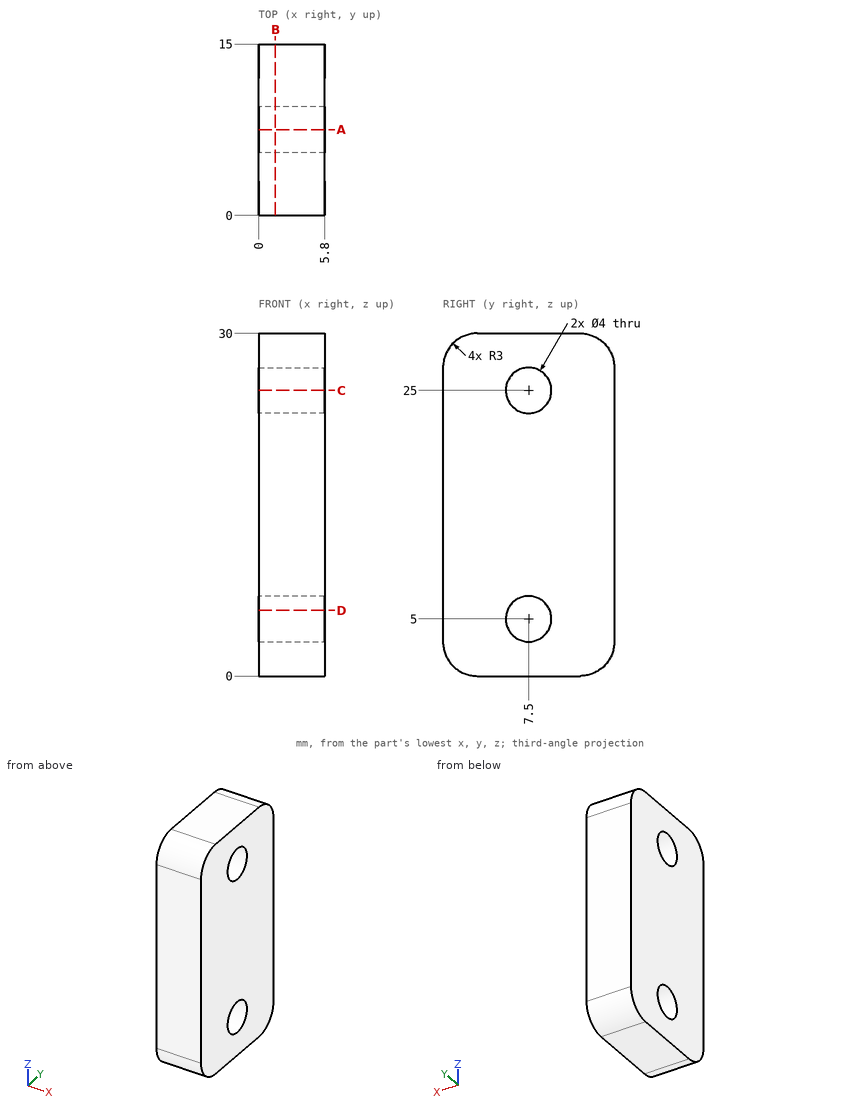
Print and shaded views of the part. All mm, measured from the part's lowest x, y and z. Round coordinates to 2 decimals unless told otherwise and drop trailing zeros. Loops run counter-clockwise (first coordinate to the right, second up) from the corner with the lowest first, then second, coordinate; pieces in that order, holes last. Notation, with made-up numbers: (7, 46) -> (65, 46) arc R20 ccw to (65, 71) -> close; hole circle Ø2 at (34, 47.5). An arc over 180 degrees is marked (long way). Use CSV: the item, a comma, the result in double quotes. Start each with the question number.
1) Wall check: L1, parallel to Y at x = 1.45, z = 5; L2, parallel to Z at x = 1.1, y = 9; L3, parallel to Z at x = 3.75, y = 6.5. Give the ranges that are in metal, low to high. Write a range as [from, to].
2) Cut at A-A, the plane y = 7.5. Write the cut outline in (x, z).
3) Cut at D-D, the plane z = 5.75. Write the cut outline in (x, y).
4) Cut at B-B, the plane x = 1.45. Write the cut outline in (y, z), plus the area to 3 significant figures.
5) Cut at C-C, the plane z = 25. Write the cut outline in (x, y), plus the area to 3 significant figures.
Determined:
1,L1,"y = [0, 5.5], [9.5, 15]"
1,L2,"z = [0, 3.68], [6.32, 23.68], [26.32, 30]"
1,L3,"z = [0, 3.27], [6.73, 23.27], [26.73, 30]"
2,outline,"(0, 0) -> (5.8, 0) -> (5.8, 3) -> (0, 3) -> close; (0, 7) -> (5.8, 7) -> (5.8, 23) -> (0, 23) -> close; (0, 27) -> (5.8, 27) -> (5.8, 30) -> (0, 30) -> close"
3,outline,"(0, 0) -> (5.8, 0) -> (5.8, 5.65) -> (0, 5.65) -> close; (0, 9.35) -> (5.8, 9.35) -> (5.8, 15) -> (0, 15) -> close"
4,outline,"(0, 3) arc R3 ccw to (3, 0) -> (12, 0) arc R3 ccw to (15, 3) -> (15, 27) arc R3 ccw to (12, 30) -> (3, 30) arc R3 ccw to (0, 27) -> close; hole circle Ø4 at (7.5, 5); hole circle Ø4 at (7.5, 25)"
4,area,"417 mm2"
5,outline,"(0, 0) -> (5.8, 0) -> (5.8, 5.5) -> (0, 5.5) -> close; (0, 9.5) -> (5.8, 9.5) -> (5.8, 15) -> (0, 15) -> close"
5,area,"63.8 mm2"
